Geometry: final body of the model. Coordinates: model frame, mm. Coordinates: 2 decimals unless noted, no trailing zeros. Write each loop counter-clockwise with the first axis right and the second up, starting at its lowest first coordinate (ties: lowest second). Pieces come first, ordered by that corner, then holes. Notation, with made-up numbers: (72.5, 54) - (116.5, 54) arc R10 ccw to (116.5, 59) - close; hole circle Ø1 at (-24.75, -3.75). An arc over 180 degrees is marked (long way). Answer as a JSON object with one key per item and string values. Group by question number.
Item 1: Section C-C on x = 3. Return loops of the section in (y, z), and give its area (4 significant figures).
Item 2: Line query: line 1 along Y through (x, z) = (44, 0.45); line 2 along Z through (x, y) = (34, -0.5); line 3 along Y through (x, z) = (13, 0.25). Output: solid intervals per line, ascending. Write a range as from..to.
Item 3: Section B-B on y = -4.25. State how many separate pieces and enclosed holes the cut face has, and give its area (3 significant figures).
Item 4: Section A-A on x = 32.5. Return loops of the section in (y, z).
Item 5: First-contact query: pin 1 Ø0.6 at (y, z) = (-1.5, 1) entering from -X (3 decimals). Flat tip, straight axial feed; report the tip coordinate or a pass-through.
Item 6: Section D-D on y = 3. Return loops of the section in (x, z), and give its area (3 significant figures).
```python
from build123d import *

# Parameters (mm, degrees)
BOSS_EXTRUDE1_DEPTH     = 0.38
BOSS_EXTRUDE2_DEPTH     = 0.38
SKETCH3_W               = 4.25
SKETCH3_H               = 0.5
BOSS_EXTRUDE3_DEPTH     = 0.75
LPATTERN1_COUNT         = 6
LPATTERN1_PITCH         = 10
CUT_EXTRUDE1_DEPTH      = 57.274439135
CUT_EXTRUDE1_DEPTH_BACK = 57.274439135
SKETCH4_W               = 2
SKETCH4_H               = 2.5


with BuildPart() as part:
    # Sketch1 → Boss-Extrude1 (new body)
    with BuildSketch(Plane.XY):
        Polygon((0, 0), (0, -2), (1.25, -2), (1.25, -5.5), (4.75, -5.5), (4.75, -2), (11.25, -2), (11.25, -5.5), (14.75, -5.5), (14.75, -2), (21.25, -2), (21.25, -5.5), (24.75, -5.5), (24.75, -2), (31.25, -2), (31.25, -5.5), (34.75, -5.5), (34.75, -2), (41.25, -2), (41.25, -5.5), (44.75, -5.5), (44.75, -2), (51.25, -2), (51.25, -5.5), (54.75, -5.5), (54.75, -2), (56, -2), (56, 0), align=None)
    extrude(amount=BOSS_EXTRUDE1_DEPTH)

    # Sketch2 → Boss-Extrude2 (add)
    with BuildSketch(Plane.XY.offset(0.38)):
        Polygon((23, 0), (23, 4), (33, 4), (33, 0), (31, 0), (31, 2), (25, 2), (25, 0), align=None)
    extrude(amount=-BOSS_EXTRUDE2_DEPTH)

    # Sketch3 → Boss-Extrude3 (add)
    with BuildSketch(Plane.XY.offset(0.38)):
        with Locations((3, -1.55)):
            Rectangle(SKETCH3_W, SKETCH3_H)
    boss_extrude3 = extrude(amount=BOSS_EXTRUDE3_DEPTH)

    # LPattern1: Boss-Extrude3 ×6
    with Locations(*[(i * LPATTERN1_PITCH, 0, 0) for i in range(1, LPATTERN1_COUNT)]):
        add(boss_extrude3)

    # Sketch4 → Cut-Extrude1 (cut, two sides: drawn at the far end of the back side and taken through both)
    with BuildSketch(Plane.XY.offset(0.38).offset(-CUT_EXTRUDE1_DEPTH_BACK)):
        with Locations((3, -4.25)):
            Rectangle(SKETCH4_W, SKETCH4_H)
        with Locations((13, -4.25)):
            Rectangle(SKETCH4_W, SKETCH4_H)
        with Locations((23, -4.25)):
            Rectangle(SKETCH4_W, SKETCH4_H)
        with Locations((33, -4.25)):
            Rectangle(SKETCH4_W, SKETCH4_H)
        with Locations((43, -4.25)):
            Rectangle(SKETCH4_W, SKETCH4_H)
        with Locations((53, -4.25)):
            Rectangle(SKETCH4_W, SKETCH4_H)
    extrude(amount=CUT_EXTRUDE1_DEPTH + CUT_EXTRUDE1_DEPTH_BACK, mode=Mode.SUBTRACT)


solid = part.part
```
Checks:
{
 "1": {"outline": "(-3, 0) - (0, 0) - (0, 0.38) - (-1.3, 0.38) - (-1.3, 1.13) - (-1.8, 1.13) - (-1.8, 0.38) - (-3, 0.38) - close", "area": "1.515 mm^2"},
 "2": {"line 1": "-1.8..-1.3", "line 2": "0..0.38", "line 3": "-3..0"},
 "3": {"separate pieces": "12", "enclosed holes": "0", "area": "3.42 mm^2"},
 "4": {"outline": "(-3, 0) - (4, 0) - (4, 0.38) - (-1.3, 0.38) - (-1.3, 1.13) - (-1.8, 1.13) - (-1.8, 0.38) - (-3, 0.38) - close"},
 "5": {"pin 1": "x = 0.875"},
 "6": {"outline": "(23, 0) - (33, 0) - (33, 0.38) - (23, 0.38) - close", "area": "3.80 mm^2"}
}
